Autodesk Inventor part; units mm, degrees
ref_plane "YZ Plane" through (0, 0, 0) normal (1, 0, 0) x (0, 1, 0)
ref_plane "XZ Plane" through (0, 0, 0) normal (0, 1, 0) x (-1, 0, 0)
ref_plane "XY Plane" through (0, 0, 0) normal (0, 0, 1) x (1, 0, 0)
sketch "Skizze1" plane through (0, 0, 0) normal (0, 1, 0) x (-1, 0, 0)
  line L0 (0, 0) -> (6, 0)
  line L1 (6, 0) -> (6, -57)
  line L2 (3, -60) -> (3, -60)
  line L3 (0, -57) -> (0, 0)
  arc A0 (3, -60) -> (6, -57) centre (3, -57) ccw
  arc A1 (0, -57) -> (3, -60) centre (3, -57) ccw
  line L4 (1, -1) -> (5, -1)
  line L5 (5, -1) -> (5, -5)
  line L6 (5, -5) -> (1, -5)
  line L7 (1, -5) -> (1, -1)
  point P0 (6, -60)
  point P1 (0, -60)
  point P2 (3, -60)
  dimension "d0" = 6
  dimension "d1" = 60
  dimension "d2" = 3
  dimension "d3" = 4
  dimension "d4" = 4
extrude "Extrusion1" add sketch "Skizze1" along normal blind 2
equation "\"Biegeradius\" = Stärke"
equation "\"BreiteBiegungsfreistellung\" = Stärke"
equation "\"TiefeBiegungsfreistellung\" = 0.5 * Stärke"
equation "\"GrößeEckenfreistellung\" = 4 * Stärke"
equation "\"MinimalRest\" = 2 * Stärke"
equation "\"Übergangsradius\" = Biegeradius"
equation "\"JacobiRadiusGröße\" = Biegeradius"
equation "\"Abstandsgröße\" = Stärke"
properties part number "V3_O4"
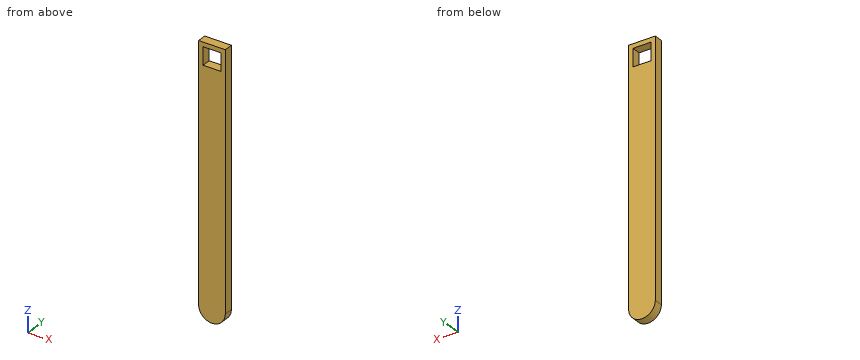
Can you work these out from the model? Positions are in its coordinate system, mm. Round coordinates to 2 decimals unless told otherwise and drop trailing zeros. Loops run counter-clockwise (first coordinate to the right, second up) from the corner with the lowest first, then second, coordinate; pieces in that order, holes last. Notation, with made-up numbers: M 24.25,9 L 61.25,9 A8 ccw 61.25,22 Z; hole C -11.5,43 d4. An arc over 180 degrees is marked long. Answer in a Markdown table with one row per item.
1. Please list where these lines run through material, in increasing order: line 1 (X direction, y = 0.4, z = -2.5); line 2 (Z direction, x = -3.25, y = 1); line 3 (Z direction, x = -4.4, y = 0.85). Write a range as from..to.
Established:
| item | result |
|---|---|
| line 1 | -6..-5, -1..0 |
| line 2 | -59.99..-5, -1..0 |
| line 3 | -59.65..-5, -1..0 |
2. If we section it at C-C, the plane z = -3.5: Please give me the cut outline in (x, y), plus the area to 3 significant figures.
Established:
| item | result |
|---|---|
| outline | M -6,0 L -5,0 L -5,2 L -6,2 Z; M -1,0 L 0,0 L 0,2 L -1,2 Z |
| area | 4.00 mm² |
3. If we section it at A-A, the plane x = -3: Please give me the cut outline in (y, z).
Established:
| item | result |
|---|---|
| outline | M 0,-60 L 2,-60 L 2,-5 L 0,-5 Z; M 0,-1 L 2,-1 L 2,0 L 0,0 Z |
4. If we section it at B-B, the plane y = 0.95: Please give me the cut outline in (x, z).
Established:
| item | result |
|---|---|
| outline | M -6,-57 A3 ccw 0,-57 L 0,0 L -6,0 Z; hole M -5,-5 L -1,-5 L -1,-1 L -5,-1 Z |
